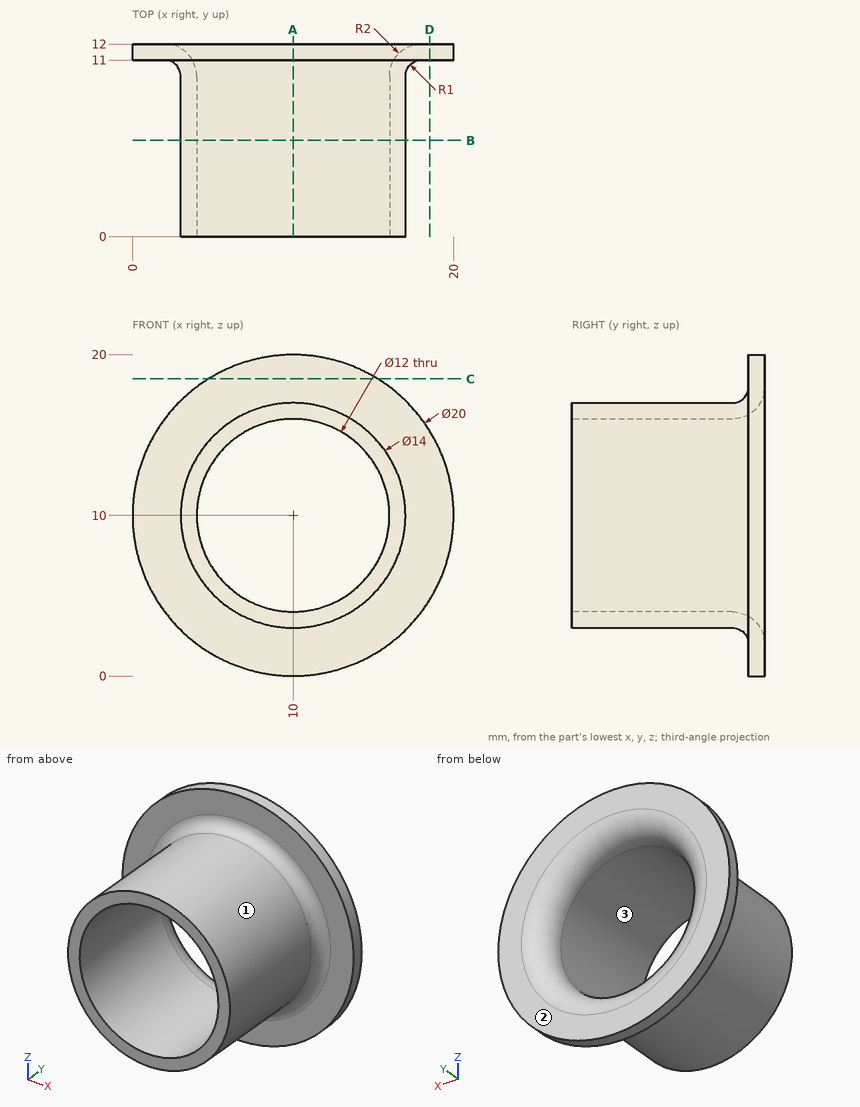
For this review, use the dimensioned drawing (mm, ordinates from the lowest corner) and the shaded views. Coordinates: 2 decimals unless noted, no trailing zeros. Loops run counter-clockwise (first coordinate to the right, second up) from the corner with the lowest first, then second, coordinate; pieces in that order, holes last.
1. Insertion check: P1, Ø1, axis at x = 10, y = 9, coming from the -Z side; P2, Ø4, axis at x = 8, y = 10, coming from the +Z side; P3, Ø2, axis at y = 3, z = 15.5, coming from the +X side. Each pin has a flat end and moves straight along its axis. Give the tip position at first contact, or say it passes through.
2. Add section C-C, the plane z = 18.5. Give the boundary of the cut face in (x, y), then the cut area to 3 significant figures.
3. Add section A-A, the plane x = 10. Give the boundary of the cut face in (y, z).
4. Add section D-D, the plane x = 18.5. Give the boundary of the cut face in (y, z), then the cut area to 3 significant figures.
5. Add section B-B, the plane y = 6. Give the boundary of the cut face in (x, z), then the cut area to 3 significant figures.
6. Mouldability with a two-part tool opening along Z and no side actions: class the marked faces 1, 2 and 3 as +Z half, -Z half, draft (parallel to the pull), parting line (faces both ways), or undercut.
7. For line 1 (X direction, y = 6.75, z = 10); line 2 (Y direction, x = 17, z = 14.5); line 3 (Z direction, x = 5.5, y = 2.25), list the stretches that pass through material, from the lowest coordinate up.
Result:
1. P1: stops at z = 3
1. P2: stops at z = 20
1. P3: stops at x = 15.36
2. outline: (4.73, 11) - (15.27, 11) - (15.27, 12) - (4.73, 12) - close
2. area: 10.5 mm2
3. outline: (0, 3) - (10, 3) arc R1 cw to (11, 2) - (11, 0) - (12, 0) - (12, 2) arc R2 ccw to (10, 4) - (0, 4) - close; (0, 16) - (10, 16) arc R2 ccw to (12, 18) - (12, 20) - (11, 20) - (11, 18) arc R1 cw to (10, 17) - (0, 17) - close
4. outline: (11, 4.73) - (12, 4.73) - (12, 15.27) - (11, 15.27) - close
4. area: 10.5 mm2
5. outline: circle Ø14 at (10, 10); hole circle Ø12 at (10, 10)
5. area: 40.8 mm2
6. face 1: parting line
6. face 2: draft
6. face 3: undercut
7. line 1: x = 3 to 4, 16 to 17
7. line 2: y = 11 to 12
7. line 3: z = 4.64 to 6.03, 13.97 to 15.36
